```python
from build123d import *

# Parameters (mm, degrees)
SKETCH1_R                  = 2.25
SKETCH1_R_2                = 1.725
BASE_FLANGE1_DEPTH         = 1.5748
SKETCHED_START             = 77.296428764
SKETCHED_BEND1_OUTLINE_W   = 45
SKETCHED_BEND1_OUTLINE_H   = 1.5748
SKETCHED_BEND1_DEPTH       = 63.903571236
SKETCHED_START_2           = 74.388620508
SKETCHED_BEND1_2_OUTLINE_W = 45
SKETCHED_BEND1_2_OUTLINE_H = 64.865020508
SKETCHED_BEND1_2_OUTLINE_R = 1.725
SKETCHED_BEND1_2_DEPTH     = 3.2512
SKETCHED_START_3           = -22.5
SKETCHED_BEND1_3_DEPTH     = 45
FILLET1_R                  = 5


with BuildPart() as part:
    # Base-Flange1: sheet metal written as solids
    # Sketch1 → Base-Flange1 (new body)
    with BuildSketch(Plane.XY):
        with BuildLine():
            Line((0, -22.5), (141.2, -22.5))
            Line((141.2, -22.5), (141.2, 22.5))
            Line((141.2, 22.5), (0, 22.5))
            ThreePointArc((0, 22.5), (-22.5, 0), (0, -22.5))
        make_face()
        with Locations((9.25, 16.02146997)):
            Circle(SKETCH1_R, mode=Mode.SUBTRACT)
        with Locations((18.5, 0)):
            Circle(SKETCH1_R, mode=Mode.SUBTRACT)
        with Locations((9.25, -16.02146997)):
            Circle(SKETCH1_R, mode=Mode.SUBTRACT)
        with Locations((-9.25, -16.02146997)):
            Circle(SKETCH1_R, mode=Mode.SUBTRACT)
        with Locations((-18.5, 0)):
            Circle(SKETCH1_R, mode=Mode.SUBTRACT)
        with Locations((-9.25, 16.02146997)):
            Circle(SKETCH1_R, mode=Mode.SUBTRACT)
        with Locations((121.2, 20)):
            Circle(SKETCH1_R_2, mode=Mode.SUBTRACT)
        with Locations((136.2, 20)):
            Circle(SKETCH1_R_2, mode=Mode.SUBTRACT)
        with Locations((136.2, -20)):
            Circle(SKETCH1_R_2, mode=Mode.SUBTRACT)
        with Locations((121.2, -20)):
            Circle(SKETCH1_R_2, mode=Mode.SUBTRACT)
    extrude(amount=-BASE_FLANGE1_DEPTH)

    # Sketched Bend1: read off the stored shape, not the designer's step
    # Sketched Bend1 outline → Sketched Bend1 (cut)
    with BuildSketch(Plane.YZ.offset(SKETCHED_START)):
        with Locations((0, -0.7874)):
            Rectangle(SKETCHED_BEND1_OUTLINE_W, SKETCHED_BEND1_OUTLINE_H)
    extrude(amount=SKETCHED_BEND1_DEPTH, mode=Mode.SUBTRACT)

    # Sketched Bend1 2 outline → Sketched Bend1 2 (add)
    with BuildSketch(Plane.YZ.offset(SKETCHED_START_2)):
        with Locations((0, 32.432510254)):
            Rectangle(SKETCHED_BEND1_2_OUTLINE_W, SKETCHED_BEND1_2_OUTLINE_H)
        with Locations((-20, 44.865020508)):
            Circle(SKETCHED_BEND1_2_OUTLINE_R, mode=Mode.SUBTRACT)
        with Locations((-20, 59.865020508)):
            Circle(SKETCHED_BEND1_2_OUTLINE_R, mode=Mode.SUBTRACT)
        with Locations((20, 44.865020508)):
            Circle(SKETCHED_BEND1_2_OUTLINE_R, mode=Mode.SUBTRACT)
        with Locations((20, 59.865020508)):
            Circle(SKETCHED_BEND1_2_OUTLINE_R, mode=Mode.SUBTRACT)
    extrude(amount=SKETCHED_BEND1_2_DEPTH)

    # Sketched Bend1 3 outline → Sketched Bend1 3 (cut)
    with BuildSketch(Plane(origin=(0, 0, 0), x_dir=(1, 0, 0), z_dir=(0, 1, 0)).offset(SKETCHED_START_3)):
        with BuildLine():
            ThreePointArc((74.388620508, 1.5748), (76.687566075, 0.622545567), (77.639820508, -1.6764))
            Line((77.639820508, -1.6764), (77.639820508, 0))
            Line((77.639820508, 0), (77.296428764, 0))
            Line((77.296428764, 0), (77.296428764, 1.5748))
            Line((77.296428764, 1.5748), (74.388620508, 1.5748))
        make_face()
        with BuildLine():
            Line((76.065020508, -64.865020508), (76.065020508, -1.6764))
            ThreePointArc((76.065020508, -1.6764), (75.574014316, -0.491006192), (74.388620508, 0))
            Line((74.388620508, 0), (74.388620508, -64.865020508))
            Line((74.388620508, -64.865020508), (76.065020508, -64.865020508))
        make_face()
    extrude(amount=SKETCHED_BEND1_3_DEPTH, mode=Mode.SUBTRACT)

    # Fillet1
    fillet1_edges = [part.edges().sort_by_distance(p)[0] for p in [
        (76.852420508, 22.5, 64.865020508),
        (76.852420508, -22.5, 64.865020508),
    ]]
    fillet(fillet1_edges, radius=FILLET1_R)


solid = part.part
```
Input: part model. Units: mm. Frame: model coordinates. A direction names the side the tool comes from. Give positions to 0.01 mm unless a question says otherwise; leave off trailing zeros. Order: outer loops, then holes, each group sorted by start corner. A loop starts at its lowest first (then second) coordinate and runs counter-clockwise, first axis right, second up. Notation, with made-up numbers: M 44,13 L 64,13 A14 cw 64,23 Z; hole C 11,44 d1. An arc over 180 degrees is marked long. Return JSON: item names as keys, results as strings.
Item 1: Cut plane B-B (y = 0). Return loops of the section in (x, z).
Solutions:
{"outline": "M -22.5,-1.57 L -20.75,-1.57 L -20.75,0 L -22.5,0 Z; M -16.25,-1.57 L 16.25,-1.57 L 16.25,0 L -16.25,0 Z; M 20.75,-1.57 L 74.39,-1.57 A3.25 ccw 77.64,1.68 L 77.64,64.87 L 76.07,64.87 L 76.07,1.68 A1.68 cw 74.39,0 L 20.75,0 Z"}
Item 2: Cut plane D-D (y = -10). Return loops of the section in (x, z), then the cut area to 3 significant figures.
Solutions:
{"outline": "M -20.16,-1.57 L 74.39,-1.57 A3.25 ccw 77.64,1.68 L 77.64,64.87 L 76.07,64.87 L 76.07,1.68 A1.68 cw 74.39,0 L -20.16,0 Z", "area": "254 mm^2"}
Item 3: Cut plane A-A (x = 9.25). Return loops of the section in (y, z), then the cut area to 3 significant figures.
Solutions:
{"outline": "M -22.5,-1.57 L -18.27,-1.57 L -18.27,0 L -22.5,0 Z; M -13.77,-1.57 L 13.77,-1.57 L 13.77,0 L -13.77,0 Z; M 18.27,-1.57 L 22.5,-1.57 L 22.5,0 L 18.27,0 Z", "area": "56.7 mm^2"}
Item 4: Cut plane C-C (x = -18.5). Return loops of the section in (y, z), then the cut area to 3 significant figures.
Solutions:
{"outline": "M -12.81,-1.57 L -2.25,-1.57 L -2.25,0 L -12.81,0 Z; M 2.25,-1.57 L 12.81,-1.57 L 12.81,0 L 2.25,0 Z", "area": "33.2 mm^2"}
Item 5: Ray query, probe 1 along Y at (x, z) = (9.25, -1.15); probe 2 along X at (y, z) = (-4.5, 15.5); probe 3 along Z at (x, y) = (43, -4.5). Return the intervals inside material, ascending.
Solutions:
{"probe 1": "-22.5 to -18.27, -13.77 to 13.77, 18.27 to 22.5", "probe 2": "76.07 to 77.64", "probe 3": "-1.57 to 0"}
Item 6: Pull-direction query (Z, two-part tool) for faces 1 (the cylindrical face through (76.841, -20.225, 61.575)), 2 (the cylindrical face through (76.863, -21.074, 63.361)), 3 (the flat face through (39, -22.5, -1)), 4 (the cylindrical face through (76.66, -0.32, -0.65)); classes: +Z half, -Z half, draft (parallel to the pull), parting line (faces both ways), or undercut.
Solutions:
{"face 1": "undercut", "face 2": "+Z half", "face 3": "draft", "face 4": "-Z half"}
Item 7: Access query for faces 5 (the cylindrical face through (76.841, -20.225, 46.575)), 6 (the flat face through (76.065, 0, 34)). Directions: +Z, -Z, +X, -X, +Y, -Y. A direction counts if a zero-diameter tool reaches every point of the face in a straight line with its end or side. Return the directions, or none.
Solutions:
{"face 5": "+X, -X", "face 6": "+Z, -X, +Y, -Y"}
Item 8: First-contact query: P1, Ø7, axis at x = 9.25, y = -16.02, coming from the +Z side; P2, Ø5.5, axis at y = 20, z = 44.87, coming from the -X side (3 decimals). Flat tips, straight axial feed; report the tip coordinate or a pass-through.
Solutions:
{"P1": "z = 0", "P2": "x = 76.065"}
